from build123d import *

# Parameters (mm, degrees)
SKETCH1_W                = 24.68
SKETCH1_H                = 23
BOSS_EXTRUDE1_DEPTH      = 1.55
BOSS_EXTRUDE2_DEPTH      = 6.3
BOSS_EXTRUDE2_DEPTH_BACK = 7.85
SKETCH2_W                = 24.68
SKETCH2_H                = 1
SKETCH3_W                = 24.68
SKETCH3_H                = 1
BOSS_EXTRUDE3_DEPTH      = 6.3
SKETCH4_W                = 24.68
SKETCH4_H                = 6.2
BOSS_EXTRUDE4_DEPTH      = 6.3
CUT_EXTRUDE1_DEPTH       = 29.336811747
FILLET1_R                = 0.5
FILLET2_R                = 0.6
SKETCH6_R                = 1.25
CUT_EXTRUDE2_DEPTH       = 10


with BuildPart() as part:
    # Sketch1 → Boss-Extrude1 (new body)
    with BuildSketch(Plane(origin=(0, 0, 0), x_dir=(1, 0, 0), z_dir=(0, 1, 0))):
        Rectangle(SKETCH1_W, SKETCH1_H)
    extrude(amount=BOSS_EXTRUDE1_DEPTH)

    # Sketch2 → Boss-Extrude2 (add, two sides: drawn at the far end of the back side and taken through both)
    with BuildSketch(Plane(origin=(0, 1.55, 0), x_dir=(1, 0, 0), z_dir=(0, 1, 0)).offset(-BOSS_EXTRUDE2_DEPTH_BACK)):
        with Locations((0, 11)):
            Rectangle(SKETCH2_W, SKETCH2_H)
        with Locations((0, -11)):
            Rectangle(SKETCH2_W, SKETCH2_H)
    extrude(amount=BOSS_EXTRUDE2_DEPTH + BOSS_EXTRUDE2_DEPTH_BACK)

    # Sketch3 → Boss-Extrude3 (add)
    with BuildSketch(Plane(origin=(0, 1.55, 0), x_dir=(1, 0, 0), z_dir=(0, 1, 0))):
        with Locations((0, 6.8)):
            Rectangle(SKETCH3_W, SKETCH3_H)
        with Locations((0, -6.8)):
            Rectangle(SKETCH3_W, SKETCH3_H)
    extrude(amount=BOSS_EXTRUDE3_DEPTH)

    # Sketch4 → Boss-Extrude4 (add)
    with BuildSketch(Plane(origin=(0, 1.55, 0), x_dir=(1, 0, 0), z_dir=(0, 1, 0))):
        Rectangle(SKETCH4_W, SKETCH4_H)
    extrude(amount=BOSS_EXTRUDE4_DEPTH)

    # Sketch5 → Cut-Extrude1 (cut, through all)
    with BuildSketch(Plane(origin=(12.34, 0, 0), x_dir=(0, 0, -1), z_dir=(1, 0, 0))):
        with BuildLine():
            Line((-2.1, 5.05), (-0.7, 5.05))
            Line((-0.7, 5.05), (-0.7, 3.835615759))
            ThreePointArc((-0.7, 3.835615759), (0, 1.55), (0.7, 3.835615759))
            Line((0.7, 3.835615759), (0.7, 5.05))
            Line((0.7, 5.05), (2.1, 5.05))
            Line((2.1, 5.05), (2.1, 8.15))
            Line((2.1, 8.15), (-2.1, 8.15))
            Line((-2.1, 8.15), (-2.1, 5.05))
        make_face()
    extrude(amount=-CUT_EXTRUDE1_DEPTH, mode=Mode.SUBTRACT)

    # Fillet1
    fillet1_edges = [part.edges().sort_by_distance(p)[0] for p in [
        (0, -6.3, -11.5),
        (0, -6.3, -10.5),
        (0, -6.3, 10.5),
        (0, -6.3, 11.5),
        (0, 7.85, -11.5),
        (0, 7.85, -10.5),
        (0, 7.85, -7.3),
        (0, 7.85, -6.3),
        (0, 7.85, -3.1),
        (0, 7.85, -2.1),
        (0, 7.85, 2.1),
        (0, 7.85, 3.1),
        (0, 7.85, 6.3),
        (0, 7.85, 7.3),
        (0, 7.85, 10.5),
        (0, 7.85, 11.5),
    ]]
    fillet(fillet1_edges, radius=FILLET1_R - 0.0001)  # a hair under: the kernel refuses the full size

    # Fillet2
    fillet2_edges = [part.edges().sort_by_distance(p)[0] for p in [
        (0, 3.835615759, -0.7),
        (0, 3.835615759, 0.7),
        (0, 5.05, 0.7),
        (0, 5.05, -0.7),
    ]]
    fillet(fillet2_edges, radius=FILLET2_R)

    # Sketch6 → Cut-Extrude2 (cut)
    with BuildSketch(Plane.XZ):
        with Locations(Location((7.67, 0, 0), (0, 0, 270))):
            Circle(SKETCH6_R)
    extrude(amount=-CUT_EXTRUDE2_DEPTH, mode=Mode.SUBTRACT)


solid = part.part
Geometry: final body of the model. Coordinates: model frame, mm. A direction names the side the tool comes from. Give positions to 0.01 mm unless a question says otherwise; leave off trailing zeros. Write each loop counter-clockwise with the first axis right and the second up, starting at its lowest first coordinate (ties: lowest second). Pieces come first, ordered by that corner, then holes. Notation, with made-up numbers: (70.5, -11.75) -> (90.5, -11.75) arc R26 ccw to (90.5, 22.25) -> close; hole circle Ø11 at (69.5, 29). An arc over 180 degrees is marked (long way). Answer in a Markdown table with one row per item.
(1) Set-up query: faces 1 (the cylindrical face through (7.69, 4.16, 1.25)), 2 (the flat face through (0, 0, 0)), 3 (the flat face through (0, 4, 3.1)). Return all of +Z, -Z, +X, -X, +Y, -Y with unobstructed straight access to the full face (end or side cutting, diameter ignored); none if empty.
Answers below:
| item | result |
|---|---|
| face 1 | +Y, -Y |
| face 2 | +X, -X, -Y |
| face 3 | +X, -X, +Y |
(2) Section query B-B on z = 9.5. Return loops of the section in (x, y).
Answers below:
| item | result |
|---|---|
| outline | (-12.34, 0) -> (12.34, 0) -> (12.34, 1.55) -> (-12.34, 1.55) -> close |
(3) Ray query, line 1 along Z through (x, y) = (-1, 2.8); line 2 along Z through (x, y) = (9.25, 6); line 3 along Z through (x, y) = (-7.25, -2). Return the intervals inside material, ascending. Write a range as [from, to].
Answers below:
| item | result |
|---|---|
| line 1 | [-11.5, -10.5], [-7.3, -6.3], [-3.1, -1.25], [1.25, 3.1], [6.3, 7.3], [10.5, 11.5] |
| line 2 | [-11.5, -10.5], [-7.3, -6.3], [-3.1, -2.1], [2.1, 3.1], [6.3, 7.3], [10.5, 11.5] |
| line 3 | [-11.5, -10.5], [10.5, 11.5] |
(4) Pin query (flat end, axial travel): pin 1 (3.5 mm diameter, centred on x = -2, z = 9, fed in from +Y); pin 2 (1.5 mm diameter, centred on x = -5.5, z = -5.5, fed in from -Y); pin 3 (1.6 mm diameter, centred on x = -2.5, z = -4, fed in from +Y). Return the tip coordinate at first contact, or that it passes through.
Answers below:
| item | result |
|---|---|
| pin 1 | y = 7.78 |
| pin 2 | y = 0 |
| pin 3 | y = 1.55 |
(5) Section query A-A on y = -1.5. Return loops of the section in (x, z), then the cut area to 3 significant figures.
Answers below:
| item | result |
|---|---|
| outline | (-12.34, -11.5) -> (12.34, -11.5) -> (12.34, -10.5) -> (-12.34, -10.5) -> close; (-12.34, 10.5) -> (12.34, 10.5) -> (12.34, 11.5) -> (-12.34, 11.5) -> close |
| area | 49.4 mm^2 |
(6) Draft query along Z for faces 4 (the flat face through (0, 1, 11.5)), 5 (the flat face through (0, 4, -10.5)), 6 (the cylindrical face through (-2.19, 1.55, 0.04)). Return one class per face: +Z half, -Z half, draft (parallel to the pull), parting line (faces both ways), or undercut.
Answers below:
| item | result |
|---|---|
| face 4 | +Z half |
| face 5 | undercut |
| face 6 | undercut |
